For this review, use the dimensioned drawing (mm, ordinates from the lowest corner) and the shaded views. A direction names the side the tool comes from. Round coordinates to 2 decimals unless told otherwise and drop trailing zeros. Loops run counter-clockwise (first coordinate to the right, second up) from the corner with the lowest first, then second, coordinate; pieces in that order, holes last. Notation, with made-up numbers: (84.25, 85) - (96.25, 85) arc R20 ccw to (96.25, 95) - close; hole circle Ø4 at (13.25, -27). An arc over 180 degrees is marked (long way). Use one line per item in the form item = value. Start each with the question number.
(1) Machinability: for the marked faces 5, 6, 7 and 8, which of the approach directions +Z, -Z, +X, -X, +Y, -Y give a long, thin tool a straight path to every point of the face, cutting with its end or side? Answer none if there is none.
(2) For pin 1 (8.5 mm diameter, centred on y = 6.5, z = 6.5, fed in from -X); pin 2 (2.5 mm diameter, centred on x = 55.8, z = 3.5, fed in from -Y); pin 3 (2 mm diameter, centred on x = 53, z = 19.5, fed in from +Y); pin 4 (5.5 mm diameter, centred on y = 11.5, z = 6, fed in from +X), all flat-tipped, find the tip position at first contact; note any pin that passes through.
(3) We need section C-C, the plane x = 43.5. Write out the cut boundary in (y, z).
(4) We need section D-D, the plane y = 7. Write out the cut boundary in (x, z).
(5) We need section A-A, the plane z = 26.5. Write out the cut boundary in (x, y), then the cut area to 3 significant figures.
(6) The part is to be moulded in two halves that separate along X. For the marked faces 1, 2, 3 and 4, say which applies: released by +X, released by -X, zero draft, split by the parting line, or undercut.
(7) Wall thickness on probe 1 along X at (y, z) = (8, 2); probe 2 along Y at (x, z) = (15.8, 2); probe 3 along X at (y, z) = (1.5, 4.5) (1 decimal): over which ranges is each line inside the solid? List them lowest first. Write a range as [from, to].
(8) We need section B-B, the plane y = 1. Give the number of separate pieces and of enclosed holes in the cut face, then the cut area to 3 significant figures.
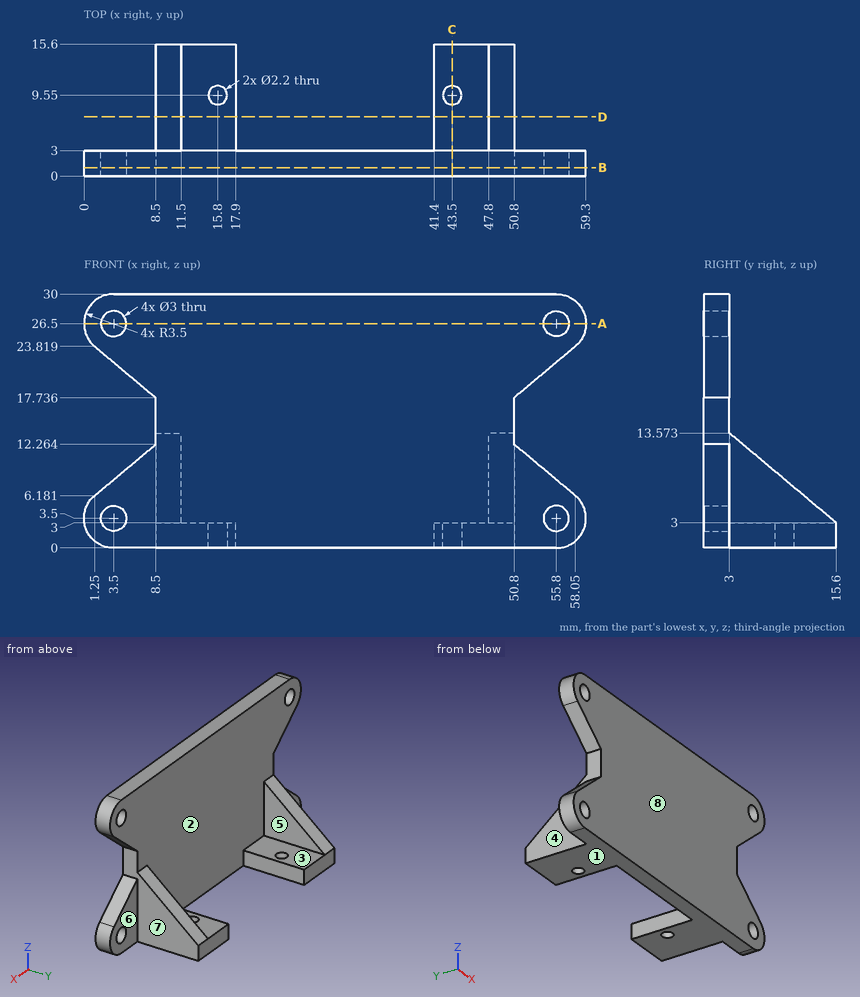
Data:
q1.face_5 = +Z, +Y
q1.face_6 = +Z, -Z, +X, +Y
q1.face_7 = +X, +Y
q1.face_8 = +Z, -Z, +X, -X, -Y
q2.pin_1 = 0.05
q2.pin_2 = through
q2.pin_3 = 3
q2.pin_4 = 50.8
q3.outline = (0, 0) - (8.45, 0) - (8.45, 3) - (3, 3) - (3, 30) - (0, 30) - close; (10.65, 0) - (15.6, 0) - (15.6, 3) - (10.65, 3) - close
q4.outline = (8.5, 0) - (17.9, 0) - (17.9, 3) - (11.5, 3) - (11.5, 10.22) - (8.5, 10.22) - close; (41.4, 0) - (50.8, 0) - (50.8, 10.22) - (47.8, 10.22) - (47.8, 3) - (41.4, 3) - close
q5.outline = (0, 0) - (2, 0) - (2, 3) - (0, 3) - close; (5, 0) - (54.3, 0) - (54.3, 3) - (5, 3) - close; (57.3, 0) - (59.3, 0) - (59.3, 3) - (57.3, 3) - close
q5.area = 160 mm^2
q6.face_1 = zero draft
q6.face_2 = undercut
q6.face_3 = undercut
q6.face_4 = released by -X
q7.probe_1 = [8.5, 17.9], [41.4, 50.8]
q7.probe_2 = [0, 8.45], [10.65, 15.6]
q7.probe_3 = [0.1, 2.4], [4.6, 54.7], [56.9, 59.2]
q8.separate_pieces = 1
q8.enclosed_holes = 4
q8.area = 1,520 mm^2
